from build123d import *

# Parameters (mm, degrees)
BOSS_EXTRUDE1_DEPTH = 3
BOSS_EXTRUDE1_TAPER = 20
CUT_EXTRUDE1_DEPTH  = 42.509035161


with BuildPart() as part:
    # Sketch1 → Boss-Extrude1 (new body)
    with BuildSketch(Plane.XY):
        with BuildLine():
            Line((-28, -25), (28, -25))
            ThreePointArc((28, -25), (31.535533906, -23.535533906), (33, -20))
            Line((33, -20), (33, 20))
            ThreePointArc((33, 20), (31.535533906, 23.535533906), (28, 25))
            Line((28, 25), (-28, 25))
            ThreePointArc((-28, 25), (-31.535533906, 23.535533906), (-33, 20))
            Line((-33, 20), (-33, -20))
            ThreePointArc((-33, -20), (-31.535533906, -23.535533906), (-28, -25))
        make_face()
    extrude(amount=BOSS_EXTRUDE1_DEPTH, taper=BOSS_EXTRUDE1_TAPER)

    # Sketch2 → Cut-Extrude1 (cut, through all)
    with BuildSketch(Plane.XY.offset(3)):
        with BuildLine():
            Line((-28, -23), (28, -23))
            ThreePointArc((28, -23), (30.121320344, -22.121320344), (31, -20))
            Line((31, -20), (31, 20))
            ThreePointArc((31, 20), (30.121320344, 22.121320344), (28, 23))
            Line((28, 23), (-28, 23))
            ThreePointArc((-28, 23), (-30.121320344, 22.121320344), (-31, 20))
            Line((-31, 20), (-31, -20))
            ThreePointArc((-31, -20), (-30.121320344, -22.121320344), (-28, -23))
        make_face()
    extrude(amount=-CUT_EXTRUDE1_DEPTH, mode=Mode.SUBTRACT)


solid = part.part
Source: CAD feature listing. Evaluate the final solid. Frame: model axes, mm. A direction names the side the tool comes from. Round coordinates to 2 decimals unless told otherwise and drop trailing zeros. Loops run counter-clockwise (first coordinate to the right, second up) from the corner with the lowest first, then second, coordinate; pieces in that order, holes last.
Q1. Section C-C, the plane z = 1.3. Return loops of the section in (x, y), plus the area to 3 significant figures.
Q2. Ray query, line 1 (X direction, y = -17.5, z = 1.15); line 2 (X direction, y = 21.5, z = 1.25); line 3 (Y direction, x = 18, z = 0.1). Return the intervals inside material, ascending.
Q3. Section A-A, the plane y = -11. Return loops of the section in (x, z).
Q4. First-contact query: P1, Ø1, axis at x = 0, z = 1.5, coming from the -Y side; P2, Ø0.9, axis at y = 3.5, z = 1.5, coming from the -X side; P3, Ø1.5, axis at y = 0.5, z = 1, coming from the +X side. Flat tips, straight axial feed; report the tip coordinate or a pass-through.
Q5. Section B-B, the plane x = -10. Return loops of the section in (y, z), plus the area to 3 significant figures.
Q6. Mould query, pull axis Y, two halves, no side actions, for faces 3 (the face through (-30.14, -22.1, 1.52)), 4 (the face through (-32.46, -0.28, 1.48)), 5 (the face through (-31.2, -23.1, 1.5)). Classes: pulls with the +Y half, pulls with the -Y half, needs draft (parallel to the pull), parting line crosses it, or undercut.
Q7. Access query for faces 1 (the face through (-31.1, 23.2, 1.5)), 2 (the face through (0, -23, 2)). Directions: +Z, -Z, +X, -X, +Y, -Y. A direction counts if a zero-diameter tool reaches every point of the face in a straight line with its end or side. Return the directions, or none.
Solutions:
1. outline: (-32.53, -20) arc R4.53 ccw to (-28, -24.53) - (28, -24.53) arc R4.53 ccw to (32.53, -20) - (32.53, 20) arc R4.53 ccw to (28, 24.53) - (-28, 24.53) arc R4.53 ccw to (-32.53, 20) - close; hole (-31, -20) arc R3 ccw to (-28, -23) - (28, -23) arc R3 ccw to (31, -20) - (31, 20) arc R3 ccw to (28, 23) - (-28, 23) arc R3 ccw to (-31, 20) - close
1. area: 329 mm2
2. line 1: x = -32.58 to -31, 31 to 32.58
2. line 2: x = -32.29 to -30.6, 30.6 to 32.29
2. line 3: y = -24.96 to -23, 23 to 24.96
3. outline: (-33, 0) - (-31, 0) - (-31, 3) - (-31.91, 3) - close; (31, 0) - (33, 0) - (31.91, 3) - (31, 3) - close
4. P1: stops at y = -24.64
4. P2: stops at x = -32.62
4. P3: stops at x = 32.91
5. outline: (-25, 0) - (-23, 0) - (-23, 3) - (-23.91, 3) - close; (23, 0) - (25, 0) - (23.91, 3) - (23, 3) - close
5. area: 8.72 mm2
6. face 3: undercut
6. face 4: needs draft
6. face 5: pulls with the -Y half
7. face 1: +Z, -X, +Y
7. face 2: +Z, -Z
